The listing builds one solid part. Answer for the finished solid, in the listing's coordinates (mm). Face numbers are marked on the shaded views. Coordinates: 2 decimals unless noted, no trailing zeros. Write each loop counter-clockwise with the first axis right and the second up, starting at its lowest first coordinate (ties: lowest second). Pieces come first, ordered by that corner, then holes.
(1) The part is cut by section C-C on x = -18. Determine the outline of the cut face in (y, z).
(2) The part is cut by section A-A on z = 12.7. Determine the outline of the cut face in (x, y) (3 decimals), plus the area to 3 significant figures.
(3) For a pull along Y with two mould halves and no side action, classify the marked faces 1, 2, 3 and 4 as +Y half, -Y half, draft (parallel to the pull), parting line (faces both ways), or undercut.
(4) Straight lines are drawn through the part: line 1 (Y direction, x = -55, z = 4.5); line 2 (Y direction, x = -59, z = 3.75); line 3 (X direction, y = 9, z = 15.25). For each, find the intervals that lie inside material, in ascending order.
(5) Given P1, Ø6, axis at y = 4, z = 7, coming from the +X side; P2, Ø4, axis at y = 2.5, z = 17.5, coming from the -X side, each flat-ended and moving along its own axis, determine where each tip first touches the part or whether it passes through.
(6) The part is cut by section B-B on x = -35. Determine the outline of the cut face in (y, z), plus the area to 3 significant figures.
(7) The part is cut by section D-D on z = 2. Determine the outline of the cut face in (x, y) (3 decimals).
from build123d import *

# Parameters (mm, degrees)
BOSS_EXTRUDE1_DEPTH = 25.4
SKETCH3_R           = 7.62
CUT_EXTRUDE1_DEPTH  = 25.4


with BuildPart() as part:
    # Sketch2 → Boss-Extrude1 (new body)
    with BuildSketch(Plane.XY):
        with BuildLine():
            ThreePointArc((-57.912, 0), (-64.897, 6.985), (-57.912, 13.97))
            Line((-57.912, 13.97), (0, 13.97))
            Line((0, 13.97), (0, 12.7))
            Line((0, 12.7), (-57.912, 12.7))
            ThreePointArc((-57.912, 12.7), (-63.627, 6.985), (-57.912, 1.27))
            Line((-57.912, 1.27), (0, 1.27))
            Line((0, 1.27), (0, 0))
            Line((0, 0), (-57.912, 0))
        make_face()
    extrude(amount=BOSS_EXTRUDE1_DEPTH)

    # Sketch3 → Cut-Extrude1 (cut)
    with BuildSketch(Plane(origin=(0, 13.97, 0), x_dir=(1, 0, 0), z_dir=(0, 1, 0))):
        with Locations(Location((-12.65707914, -12.7, 0), (0, 0, 180))):
            Circle(SKETCH3_R)
    extrude(amount=-CUT_EXTRUDE1_DEPTH, mode=Mode.SUBTRACT)


solid = part.part
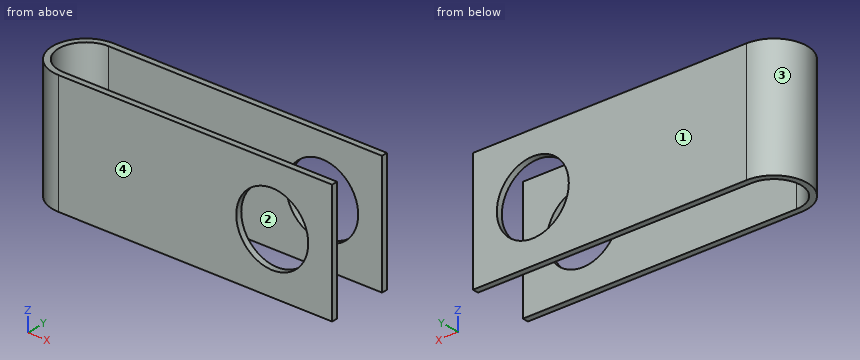
Model answer:
1. outline: (0, 0) - (1.27, 0) - (1.27, 7.27) - (0, 7.27) - close; (0, 18.13) - (1.27, 18.13) - (1.27, 25.4) - (0, 25.4) - close; (12.7, 0) - (13.97, 0) - (13.97, 7.27) - (12.7, 7.27) - close; (12.7, 18.13) - (13.97, 18.13) - (13.97, 25.4) - (12.7, 25.4) - close
2. outline: (-57.912, 0) - (-20.277, 0) - (-20.277, 1.27) - (-57.912, 1.27) arc R5.715 cw to (-57.912, 12.7) - (-20.277, 12.7) - (-20.277, 13.97) - (-57.912, 13.97) arc R6.985 ccw to start; (-5.037, 0) - (0, 0) - (0, 1.27) - (-5.037, 1.27) - close; (-5.037, 12.7) - (0, 12.7) - (0, 13.97) - (-5.037, 13.97) - close
2. area: 134 mm2
3. face 1: +Y half
3. face 2: undercut
3. face 3: parting line
3. face 4: -Y half
4. line 1: y = 0 to 1.27, 12.7 to 13.97
4. line 2: y = 0.09 to 1.37, 12.6 to 13.88
4. line 3: x = -64.6 to -63.26
5. P1: stops at x = 0
5. P2: stops at x = -64.44
6. outline: (0, 0) - (1.27, 0) - (1.27, 25.4) - (0, 25.4) - close; (12.7, 0) - (13.97, 0) - (13.97, 25.4) - (12.7, 25.4) - close
6. area: 64.5 mm2
7. outline: (-57.912, 0) - (0, 0) - (0, 1.27) - (-57.912, 1.27) arc R5.715 cw to (-57.912, 12.7) - (0, 12.7) - (0, 13.97) - (-57.912, 13.97) arc R6.985 ccw to start
